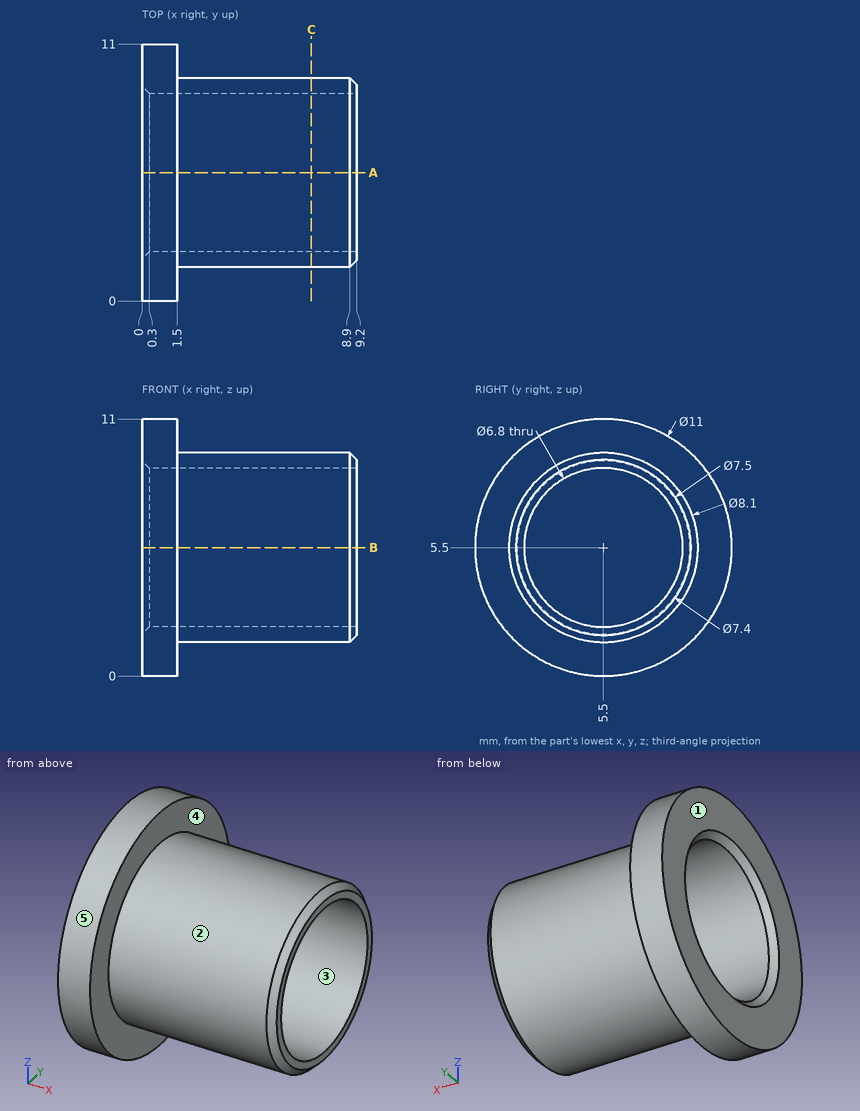
Here's the drawing with two shaded views (mm, measured from the low corner). I have some questions. A direction names the side the tool comes from. Coordinates: 2 decimals unless noted, no trailing zeros. Order: outer loops, then holes, each group sorted by start corner. A loop starts at its lowest first (then second) coordinate and runs counter-clockwise, first axis right, second up.
Item 1: I need wall thicknesses on probe 1 along Z at (x, y) = (8.5, 5.5); probe 2 along Y at (x, z) = (8.25, 4). Which ranges of each line are inside material? Lowest first, please.
Response values:
probe 1: z = 1.45 to 2.1, 8.9 to 9.55
probe 2: y = 1.74 to 2.45, 8.55 to 9.26
Item 2: If we section it at A-A, the plane y = 5.5: List the corners of the cut face in (x, z) for me, then the cut area to 3 significant figures.
Response values:
outline: (0, 0) - (1.5, 0) - (1.5, 1.45) - (8.9, 1.45) - (9.2, 1.75) - (9.2, 2.1) - (0.3, 2.1) - (0, 1.8) - close; (0, 9.2) - (0.3, 8.9) - (9.2, 8.9) - (9.2, 9.25) - (8.9, 9.55) - (1.5, 9.55) - (1.5, 11) - (0, 11) - close
area: 16.1 mm2
Item 3: If we section it at C-C, the plane x = 7.25: List the corners of the cut face in (y, z) for me.
Response values:
outline: circle Ø8.1 at (5.5, 5.5); hole circle Ø6.8 at (5.5, 5.5)
Item 4: Thinking about a two-plate mould opening in Y: for the marked faces 1, 2 and 3, which applies, pulls with the +Y half, pulls with the -Y half, needs draft (parallel to the pull), parting line crosses it, or undercut?
Response values:
face 1: needs draft
face 2: parting line crosses it
face 3: undercut
Item 5: Which directions (+Z, -Z, +X, -X, +Y, -Y) give clear straight access to the entire face, cutting with the end or side of a thin tool? Please do the marked faces 4 and 5.
Response values:
face 4: +X
face 5: +X, -X
Item 6: I'm going to push flat-ended pins straight in: pin 1 Ø5 at (x, z) = (7.5, 1.5) entering from -Y; pin 2 Ø2 at (x, z) = (8, 4) entering from -Y; pin 3 Ø5 at (x, y) = (7, 2.5) entering from -Z; pin 4 Ø5.5 at (y, z) = (5.5, 5.5) entering from +X. Where does each tip first touch, or does it pass through?
Response values:
pin 1: stops at y = 1.74
pin 2: stops at y = 1.48
pin 3: stops at z = 1.48
pin 4: passes through
